from build123d import *

# Parameters (mm, degrees)
ESQUISSE1_R        = 1.45
ESQUISSE1_W        = 2
ESQUISSE1_H        = 4
ESQUISSE1_W_2      = 6.9
ESQUISSE1_H_2      = 6.9
BOSS_EXTRU_1_DEPTH = 3


with BuildPart() as part:
    # Esquisse1 → Boss.-Extru.1 (new body)
    with BuildSketch(Plane(origin=(0, 0, 0), x_dir=(1, 0, 0), z_dir=(0, 1, 0))):
        Polygon((30.85, 0), (46.55, 0), (46.55, 25.5), (58.05, 25.5), (58.05, 0), (64.05, 0), (64.05, 25.5), (75.55, 25.5), (75.55, 0), (86, 0), (86, 76), (75.55, 76), (75.55, 50.5), (64.05, 50.5), (64.05, 76), (58.05, 76), (58.05, 50.5), (46.55, 50.5), (46.55, 76), (30.85, 76), (30.85, 50.5), (19.35, 50.5), (19.35, 76), (0, 76), (0, 57), (7, 57), (7, 19), (0, 19), (0, 0), (19.35, 0), (19.35, 25.5), (30.85, 25.5), align=None)
        with Locations(Location((16.35, 13.25, 0), (0, 0, 270))):
            Circle(ESQUISSE1_R, mode=Mode.SUBTRACT)
        with Locations(Location((78.55, 13.25, 0), (0, 0, 270))):
            Circle(ESQUISSE1_R, mode=Mode.SUBTRACT)
        with Locations(Location((78.55, 62.75, 0), (0, 0, 90))):
            Circle(ESQUISSE1_R, mode=Mode.SUBTRACT)
        with Locations(Location((16.35, 62.75, 0), (0, 0, 90))):
            Circle(ESQUISSE1_R, mode=Mode.SUBTRACT)
        with Locations((61.05, 7)):
            Rectangle(ESQUISSE1_W, ESQUISSE1_H, mode=Mode.SUBTRACT)
        with Locations((16.35, 7)):
            Rectangle(ESQUISSE1_W, ESQUISSE1_H, mode=Mode.SUBTRACT)
        with Locations((80.55, 38)):
            Rectangle(ESQUISSE1_W_2, ESQUISSE1_H_2, mode=Mode.SUBTRACT)
        with Locations((33.85, 7)):
            Rectangle(ESQUISSE1_W, ESQUISSE1_H, mode=Mode.SUBTRACT)
        with Locations((5.45, 5.45)):
            Rectangle(ESQUISSE1_W_2, ESQUISSE1_H_2, mode=Mode.SUBTRACT)
        with Locations((33.85, 21)):
            Rectangle(ESQUISSE1_W, ESQUISSE1_H, mode=Mode.SUBTRACT)
        with Locations((16.35, 21)):
            Rectangle(ESQUISSE1_W, ESQUISSE1_H, mode=Mode.SUBTRACT)
        with Locations((78.55, 7)):
            Rectangle(ESQUISSE1_W, ESQUISSE1_H, mode=Mode.SUBTRACT)
        with Locations((78.55, 21)):
            Rectangle(ESQUISSE1_W, ESQUISSE1_H, mode=Mode.SUBTRACT)
        with Locations((61.05, 21)):
            Rectangle(ESQUISSE1_W, ESQUISSE1_H, mode=Mode.SUBTRACT)
        with Locations((61.05, 55)):
            Rectangle(ESQUISSE1_W, ESQUISSE1_H, mode=Mode.SUBTRACT)
        with Locations((78.55, 55)):
            Rectangle(ESQUISSE1_W, ESQUISSE1_H, mode=Mode.SUBTRACT)
        with Locations((78.55, 69)):
            Rectangle(ESQUISSE1_W, ESQUISSE1_H, mode=Mode.SUBTRACT)
        with Locations((16.35, 55)):
            Rectangle(ESQUISSE1_W, ESQUISSE1_H, mode=Mode.SUBTRACT)
        with Locations((33.85, 55)):
            Rectangle(ESQUISSE1_W, ESQUISSE1_H, mode=Mode.SUBTRACT)
        with Locations((33.85, 69)):
            Rectangle(ESQUISSE1_W, ESQUISSE1_H, mode=Mode.SUBTRACT)
        with Locations((5.45, 70.55)):
            Rectangle(ESQUISSE1_W_2, ESQUISSE1_H_2, mode=Mode.SUBTRACT)
        with Locations((61.05, 69)):
            Rectangle(ESQUISSE1_W, ESQUISSE1_H, mode=Mode.SUBTRACT)
        with Locations((16.35, 69)):
            Rectangle(ESQUISSE1_W, ESQUISSE1_H, mode=Mode.SUBTRACT)
        with Locations((43.55, 55)):
            Rectangle(ESQUISSE1_W, ESQUISSE1_H, mode=Mode.SUBTRACT)
        with Locations((43.55, 7)):
            Rectangle(ESQUISSE1_W, ESQUISSE1_H, mode=Mode.SUBTRACT)
        with Locations((43.55, 21)):
            Rectangle(ESQUISSE1_W, ESQUISSE1_H, mode=Mode.SUBTRACT)
        with Locations((43.55, 69)):
            Rectangle(ESQUISSE1_W, ESQUISSE1_H, mode=Mode.SUBTRACT)
    extrude(amount=BOSS_EXTRU_1_DEPTH)


solid = part.part
Geometry check sheet. Reference: the model listing, model coordinates, mm. A direction names the side the tool comes from. Round coordinates to 2 decimals unless told otherwise and drop trailing zeros. Write each loop counter-clockwise with the first axis right and the second up, starting at its lowest first coordinate (ties: lowest second). Pieces come first, ordered by that corner, then holes.
Item 1: Section check D-D (z = -59). Record the boundary of the cut face in (x, y).
Determined:
outline: (0, 0) - (19.35, 0) - (19.35, 3) - (0, 3) - close; (30.85, 0) - (46.55, 0) - (46.55, 3) - (30.85, 3) - close; (58.05, 0) - (64.05, 0) - (64.05, 3) - (58.05, 3) - close; (75.55, 0) - (86, 0) - (86, 3) - (75.55, 3) - close
Item 2: Material ranges on line 1 along X through (y, z) = (1.6, -72); line 2 along X through (y, z) = (2.3, -62.75); line 3 along Z through (x, y) = (61, 2.3), recorded low to high.
Determined:
line 1: x = 0 to 2, 8.9 to 19.35, 30.85 to 46.55, 58.05 to 64.05, 75.55 to 86
line 2: x = 0 to 14.9, 17.8 to 19.35, 30.85 to 46.55, 58.05 to 64.05, 75.55 to 77.1, 80 to 86
line 3: z = -76 to -71, -67 to -57, -53 to -23, -19 to -9, -5 to 0
Item 3: Section check B-B (z = -13.25). Record the boundary of the cut face in (x, y).
Determined:
outline: (0, 0) - (14.9, 0) - (14.9, 3) - (0, 3) - close; (17.8, 0) - (19.35, 0) - (19.35, 3) - (17.8, 3) - close; (30.85, 0) - (46.55, 0) - (46.55, 3) - (30.85, 3) - close; (58.05, 0) - (64.05, 0) - (64.05, 3) - (58.05, 3) - close; (75.55, 0) - (77.1, 0) - (77.1, 3) - (75.55, 3) - close; (80, 0) - (86, 0) - (86, 3) - (80, 3) - close
Item 4: Mould release check, pull along X, two halves, no side actions. Record for faces 4 (the face through (0, 1, -67)), 5 (the face through (42, 3, -39)), 6 (the face through (17.35, 1, -69)): +X half, -X half, draft (parallel to the pull), parting line (faces both ways), or undercut.
Determined:
face 4: -X half
face 5: draft
face 6: undercut
Item 5: Access from +Z, -Z, +X, -X, +Y, -Y to the whole of each face (thin tool, end or side, straight path). Record for faces 1 (the face through (81, 1, -76)), 2 (the face through (58.05, 1, -13)), 3 (the face through (79, 1, -9)).
Determined:
face 1: -Z, +X, -X, +Y, -Y
face 2: +Z, +Y, -Y
face 3: +Y, -Y
Item 6: Section check C-C (x = 78.55). Give the number of separate pieces and of enclosed holes in the cut face, plus the area to 3 significant figures.
Determined:
separate pieces: 8
enclosed holes: 0
area: 142 mm2
Item 7: Go/stop test with flat-tipped pins: pin 1 Ø0.9 at (y, z) = (1.5, -54.5) entering from -X; pin 2 Ø12 at (x, z) = (33.5, -17) entering from -Y; pin 3 Ø2.5 at (x, z) = (78.55, -13.25) entering from -Y. Record where each tip stops, or that it passes through.
Determined:
pin 1: stops at x = 7
pin 2: stops at y = 0
pin 3: passes through
Item 8: Section check A-A (x = 16.35). Record the boundary of the cut face in (y, z), plus the area to 3 significant figures.
Determined:
outline: (0, -76) - (3, -76) - (3, -71) - (0, -71) - close; (0, -67) - (3, -67) - (3, -64.2) - (0, -64.2) - close; (0, -61.3) - (3, -61.3) - (3, -57) - (0, -57) - close; (0, -53) - (3, -53) - (3, -23) - (0, -23) - close; (0, -19) - (3, -19) - (3, -14.7) - (0, -14.7) - close; (0, -11.8) - (3, -11.8) - (3, -9) - (0, -9) - close; (0, -5) - (3, -5) - (3, 0) - (0, 0) - close
area: 163 mm2
